Source: CAD feature listing. Evaluate the final solid. Frame: model axes, mm. A direction names the side the tool comes from. Round coordinates to 2 decimals unless told otherwise and drop trailing zeros. Order: outer loops, then holes, each group sorted by start corner. A loop starts at its lowest first (then second) coordinate and runs counter-clockwise, first axis right, second up. Notation, with made-up numbers: M 77.25,4.25 L 128.25,4.25 A21 ccw 128.25,10.25 Z; hole C -28.75,-28 d2. An arc over 180 degrees is marked long. Use one line per item in the form item = value. Start each with the question number.
Q1. Pull-direction query (Y, two-part tool) for faces 6 (the flat face through (0, -23.749, 3)), 7 (the flat face through (0, 28, 1.705)), 8 (the flat face through (4, 1, 2.54)); classes: pulls with the +Y half, pulls with the -Y half, needs draft (parallel to the pull), parting line crosses it, or undercut.
Q2. Contact query for flat-ended pins moving along their axis: pin 1 (2 mm diameter, centred on y = 26, z = 2.5, fed in from +X); pin 2 (2 mm diameter, centred on y = 26, z = 3.5, fed in from -X); pin 3 (2.5 mm diameter, centred on x = -2.5, y = 26, fed in from -Z) (3 decimals). Output: stop coordinate, or through.
Q3. Section B-B (z = 1). Return the cut outline in (x, y).
Q4. Section A-A (y = 4). Return the cut outline in (x, z), plus the area to 3 significant figures.
Q5. Reachability of faces 1 (the flat face through (0, 28, 4.245)), 2 (the flat face through (-5.156, 5.202, 4.269)), 3 (the flat face through (5.08, 28, 3)), 4 (the flat face through (0, 0, 0)), 5 (the flat face through (-5.08, 28, 3)) from +Z, -Z, +X, -X, +Y, -Y: full face, straight path, thin tool, end or side. Return the list, or none.
Q6. Material intervals for probe 1 along Y at (x, z) = (3.5, 5.1); probe 2 along Y at (x, z) = (1.75, 3.8); probe 3 along Y at (x, z) = (5.75, 4.95), sorted ascending.
from build123d import *

# Parameters (mm, degrees)
SKETCH1_W           = 17.38
SKETCH1_H           = 47.498
BOSS_EXTRUDE1_DEPTH = 5.95
CUT_EXTRUDE1_DEPTH  = 3.41
SKETCH3_W           = 10.16
SKETCH3_H           = 2.54
BOSS_EXTRUDE2_DEPTH = 7.62


with BuildPart() as part:
    # Sketch1 → Boss-Extrude1 (new body)
    with BuildSketch(Plane.XY):
        Rectangle(SKETCH1_W, SKETCH1_H)
    extrude(amount=BOSS_EXTRUDE1_DEPTH)

    # Sketch2 → Cut-Extrude1 (cut)
    with BuildSketch(Plane.XY.offset(5.95)):
        with BuildLine():
            Line((7.442756003, 9.924455156), (7.491268126, 9.618455606))
            add(Edge.make_bspline(
                [(7.491268126, 9.618455606), (7.388196446, 9.466942554), (7.190794115, 9.176765567), (6.883635039, 8.77416687), (6.580334345, 8.424256906), (6.271574884, 8.117843462), (5.940370317, 7.841299159), (5.568441188, 7.578876003), (5.153754118, 7.310436522), (4.852926765, 7.147246701), (4.696223459, 7.062239856)],
                knots=[0, 0, 0, 0, 1.145964768, 2.194745584, 3.165202406, 4.03990847, 4.912501504, 5.860303535, 6.885415487, 8, 8, 8, 8], degree=3))
            add(Edge.make_bspline(
                [(4.696223459, 7.062239856), (4.499744398, 6.967232704), (4.102902364, 6.775340341), (3.474153814, 6.538191996), (2.813554004, 6.333237061), (2.120776353, 6.162580703), (1.399657714, 6.026815112), (0.651510405, 5.937381635), (-0.120298453, 5.873381172), (-0.643704604, 5.867395245), (-0.908792682, 5.86436357)],
                knots=[0, 0, 0, 0, 0.905325806, 1.828547692, 2.785348579, 3.774441141, 4.787925238, 5.828395329, 6.90015334, 8, 8, 8, 8], degree=3))
            add(Edge.make_bspline(
                [(-0.908792682, 5.86436357), (-1.183775776, 5.868319524), (-1.744155055, 5.876381236), (-2.60042752, 5.931891418), (-3.488027549, 6.016072254), (-4.088461448, 6.098524731), (-4.394202187, 6.140509505)],
                knots=[0, 0, 0, 0, 0.943008224, 1.921726389, 2.941743778, 4, 4, 4, 4], degree=3))
            Line((-4.394202187, 6.140509505), (-5.245030203, 1.177346077))
            add(Edge.make_bspline(
                [(-5.245030203, 1.177346077), (-5.099692133, 1.252367706), (-4.817426132, 1.398069757), (-4.4023402, 1.604243124), (-4.006704111, 1.790847965), (-3.632644493, 1.958676402), (-3.278177346, 2.103991861), (-2.947838119, 2.237174313), (-2.634386649, 2.343936776), (-2.239987634, 2.466535927), (-1.735943769, 2.588441657), (-1.096664304, 2.685171937), (-0.408909829, 2.752005624), (0.066252368, 2.757006699), (0.311473815, 2.759587651)],
                knots=[0, 0, 0, 0, 1.006594111, 1.95494061, 2.852161939, 3.698632082, 4.47771994, 5.20984462, 5.890144692, 6.514895121, 7.751501423, 9.076797217, 10.491395109, 12, 12, 12, 12], degree=3))
            add(Edge.make_bspline(
                [(0.311473815, 2.759587651), (0.535398839, 2.755977577), (0.974846729, 2.748892886), (1.620475428, 2.715284292), (2.237431508, 2.640791764), (2.828133868, 2.549610207), (3.391581711, 2.431161677), (3.926410539, 2.283829718), (4.436803767, 2.118613947), (4.916396667, 1.918999578), (5.371826845, 1.701125088), (5.793685602, 1.447774573), (6.191678015, 1.175540089), (6.432055206, 0.966979497), (6.550879266, 0.863883124)],
                knots=[0, 0, 0, 0, 1.209491551, 2.373600323, 3.489351857, 4.563959151, 5.600865615, 6.596587735, 7.558914106, 8.495791867, 9.400120309, 10.282627716, 11.15106276, 12, 12, 12, 12], degree=3))
            add(Edge.make_bspline(
                [(6.550879266, 0.863883124), (6.663701743, 0.742591932), (6.887885733, 0.501580172), (7.185905623, 0.107991252), (7.434808919, -0.317506707), (7.64735089, -0.762667624), (7.815411217, -1.223810977), (7.933572717, -1.692856119), (8.013981471, -2.164737406), (8.021265636, -2.481883253), (8.024901487, -2.64018489)],
                knots=[0, 0, 0, 0, 1.019710416, 2.026216391, 3.032489163, 4.05009723, 5.060530396, 6.048889042, 7.026113504, 8, 8, 8, 8], degree=3))
            add(Edge.make_bspline(
                [(8.024901487, -2.64018489), (8.020801767, -2.804619839), (8.012753023, -3.127445431), (7.943075826, -3.602494497), (7.831393213, -4.057156952), (7.67809346, -4.496086456), (7.475268481, -4.912593105), (7.231250027, -5.312871427), (6.938962553, -5.690361738), (6.716016962, -5.922311768), (6.603123092, -6.039765252)],
                knots=[0, 0, 0, 0, 1.041176999, 2.04408236, 3.034027167, 4.003470328, 4.983202096, 5.962965549, 6.968498547, 8, 8, 8, 8], degree=3))
            add(Edge.make_bspline(
                [(6.603123092, -6.039765252), (6.405699461, -6.215392151), (6.007486189, -6.569640332), (5.32662517, -7.011218259), (4.58377472, -7.392320821), (3.766799238, -7.694680543), (2.886211455, -7.939522552), (1.934509396, -8.101388624), (0.917305834, -8.210370201), (0.214760817, -8.221040232), (-0.14752551, -8.226542522)],
                knots=[0, 0, 0, 0, 0.871069273, 1.756990004, 2.669566264, 3.621983655, 4.627000268, 5.682036848, 6.804679652, 8, 8, 8, 8], degree=3))
            add(Edge.make_bspline(
                [(-0.14752551, -8.226542522), (-0.370250634, -8.222244049), (-0.816200421, -8.213637462), (-1.482946375, -8.166140654), (-2.145331954, -8.078795756), (-2.791605268, -7.961417463), (-3.403604951, -7.819259345), (-3.958712163, -7.654815969), (-4.453900955, -7.481257394), (-4.749947343, -7.333786701), (-4.890518529, -7.263763451)],
                knots=[0, 0, 0, 0, 1.095684565, 2.19382659, 3.285951729, 4.380508114, 5.423877159, 6.374492448, 7.228163105, 8, 8, 8, 8], degree=3))
            add(Edge.make_bspline(
                [(-4.890518529, -7.263763451), (-5.035629193, -7.182452627), (-5.316509414, -7.025065144), (-5.694035748, -6.740579878), (-6.019519859, -6.431088542), (-6.295032988, -6.097913353), (-6.51309252, -5.744206053), (-6.667017422, -5.373777783), (-6.766809982, -4.991418752), (-6.777243361, -4.730546951), (-6.782491355, -4.599328348)],
                knots=[0, 0, 0, 0, 1.160681474, 2.246647206, 3.291271732, 4.291304077, 5.25829909, 6.181203858, 7.085144929, 8, 8, 8, 8], degree=3))
            add(Edge.make_bspline(
                [(-6.782491355, -4.599328348), (-6.774342349, -4.453081073), (-6.75846843, -4.168197538), (-6.64211866, -3.759871717), (-6.436538728, -3.397764213), (-6.163895247, -3.081023671), (-5.833430689, -2.820020292), (-5.457625005, -2.631179544), (-5.044250192, -2.513816473), (-4.755734581, -2.501171297), (-4.606909191, -2.494648518)],
                knots=[0, 0, 0, 0, 1.038363749, 2.022688871, 2.983899271, 3.973918752, 4.974410771, 5.954403577, 6.944817285, 8, 8, 8, 8], degree=3))
            add(Edge.make_bspline(
                [(-4.606909191, -2.494648518), (-4.507163048, -2.496981892), (-4.312628946, -2.501532653), (-4.031008634, -2.552467514), (-3.765664982, -2.629947355), (-3.520661715, -2.74257489), (-3.294573312, -2.881087206), (-3.092603306, -3.045610231), (-2.914473539, -3.235149346), (-2.763280777, -3.446234353), (-2.638351732, -3.674894842), (-2.548205754, -3.918478563), (-2.494918861, -4.17535582), (-2.487384773, -4.350303052), (-2.483570852, -4.438865169)],
                knots=[0, 0, 0, 0, 1.117637543, 2.179719547, 3.199437565, 4.211008827, 5.194574363, 6.166491412, 7.123978993, 8.103677089, 9.071378429, 10.038174012, 11.006880757, 12, 12, 12, 12], degree=3))
            add(Edge.make_bspline(
                [(-2.483570852, -4.438865169), (-2.486995627, -4.527517151), (-2.493771023, -4.70290165), (-2.552315647, -4.956438553), (-2.640742431, -5.197727564), (-2.776563998, -5.418114374), (-2.939315934, -5.629950077), (-3.146823442, -5.820016584), (-3.384493352, -6.001663071), (-3.565500253, -6.100586139), (-3.659056927, -6.151716307)],
                knots=[0, 0, 0, 0, 0.968529955, 1.916089601, 2.833465673, 3.766948701, 4.736052034, 5.746774587, 6.835379905, 8, 8, 8, 8], degree=3))
            add(Edge.make_bspline(
                [(-3.659056927, -6.151716307), (-3.712593015, -6.195118685), (-3.810012219, -6.274097656), (-3.926920197, -6.402182193), (-4.001195782, -6.530313333), (-4.012238567, -6.618709273), (-4.017300302, -6.659227755)],
                knots=[0, 0, 0, 0, 1.288779764, 2.34518258, 3.241473203, 4, 4, 4, 4], degree=3))
            add(Edge.make_bspline(
                [(-4.017300302, -6.659227755), (-4.014862106, -6.693558852), (-4.009786068, -6.765032163), (-3.94889938, -6.86383505), (-3.865505152, -6.962509198), (-3.747621078, -7.0590999), (-3.59734133, -7.150700716), (-3.414668231, -7.240893328), (-3.200044936, -7.328812331), (-2.867030136, -7.443506304), (-2.414722193, -7.569316413), (-1.839757858, -7.670449008), (-1.236208093, -7.736106558), (-0.824385614, -7.744563892), (-0.613988238, -7.748884688)],
                knots=[0, 0, 0, 0, 0.326627239, 0.679999541, 1.087570525, 1.571741335, 2.136209263, 2.778409567, 3.529552134, 4.365937735, 6.165921372, 8.039005593, 9.976354196, 12, 12, 12, 12], degree=3))
            add(Edge.make_bspline(
                [(-0.613988238, -7.748884688), (-0.42349165, -7.745898893), (-0.053933814, -7.740106537), (0.480092866, -7.67864014), (0.976569924, -7.583764599), (1.432246926, -7.446925264), (1.848139012, -7.268810492), (2.227817186, -7.057803498), (2.567389934, -6.802022096), (2.864540024, -6.502050413), (3.12901858, -6.16407249), (3.352639163, -5.778648178), (3.54280588, -5.350498704), (3.699090595, -4.879386484), (3.817527637, -4.363147203), (3.901267526, -3.80421506), (3.954403228, -3.199710621), (3.96125619, -2.7821062), (3.964809902, -2.565550853)],
                knots=[0, 0, 0, 0, 1.145984371, 2.223176321, 3.230327741, 4.184709763, 5.080198491, 5.948392179, 6.792829292, 7.629197606, 8.482744051, 9.368637587, 10.303560962, 11.297831961, 12.351033038, 13.487071465, 14.696881343, 16, 16, 16, 16], degree=3))
            add(Edge.make_bspline(
                [(3.964809902, -2.565550853), (3.959937282, -2.315186172), (3.95054273, -1.832475769), (3.854905269, -1.138827256), (3.705638698, -0.502736617), (3.487857452, 0.072698671), (3.212336232, 0.590456281), (2.869977731, 1.042931556), (2.464404193, 1.430095093), (1.998885296, 1.746615006), (1.483054716, 1.997270407), (0.925314836, 2.181919986), (0.322799369, 2.28608044), (-0.091155302, 2.300584907), (-0.304256986, 2.308051731)],
                knots=[0, 0, 0, 0, 1.224131662, 2.360161531, 3.418424534, 4.414143726, 5.361687872, 6.278160415, 7.177748908, 8.092603741, 9.020660508, 9.975155306, 10.957620613, 12, 12, 12, 12], degree=3))
            add(Edge.make_bspline(
                [(-0.304256986, 2.308051731), (-0.585965965, 2.299911613), (-1.136361477, 2.284007669), (-1.811836605, 2.167686698), (-2.337007345, 2.039517007), (-2.732310337, 1.908362031), (-3.140497373, 1.762367668), (-3.553566201, 1.578877843), (-3.981742925, 1.379844177), (-4.417153582, 1.143324516), (-4.874022359, 0.893907905), (-5.176248262, 0.706169561), (-5.330859345, 0.6101274)],
                knots=[0, 0, 0, 0, 1.569199768, 3.065860781, 3.809147302, 4.580990623, 5.38603441, 6.224540817, 7.099163695, 8.017256459, 8.985678849, 10, 10, 10, 10], degree=3))
            Line((-5.330859345, 0.6101274), (-5.827175687, 0.6101274))
            Line((-5.827175687, 0.6101274), (-4.465104521, 9.924455156))
            add(Edge.make_bspline(
                [(-4.465104521, 9.924455156), (-4.315984039, 9.880431687), (-4.028541468, 9.795572662), (-3.610488685, 9.680706455), (-3.217546123, 9.59555299), (-2.963853205, 9.550545578), (-2.841814227, 9.528894762)],
                knots=[0, 0, 0, 0, 1.115879267, 2.150953381, 3.110516124, 4, 4, 4, 4], degree=3))
            add(Edge.make_bspline(
                [(-2.841814227, 9.528894762), (-2.510146411, 9.477884697), (-1.830201619, 9.373310099), (-0.775608412, 9.285032005), (0.332929285, 9.21530606), (1.09127166, 9.210452917), (1.479496486, 9.207968405)],
                knots=[0, 0, 0, 0, 0.928037139, 1.90254824, 2.926233227, 4, 4, 4, 4], degree=3))
            add(Edge.make_bspline(
                [(1.479496486, 9.207968405), (1.857705195, 9.211620808), (2.587136827, 9.218665008), (3.650367069, 9.270738299), (4.655930506, 9.361259539), (5.618408289, 9.504787441), (6.545008139, 9.689890411), (7.146144347, 9.846956071), (7.442756003, 9.924455156)],
                knots=[0, 0, 0, 0, 1.129737635, 2.178866713, 3.179008279, 4.144335706, 5.084381125, 6, 6, 6, 6], degree=3))
        make_face()
    extrude(amount=-CUT_EXTRUDE1_DEPTH, mode=Mode.SUBTRACT)

    # Sketch3 → Boss-Extrude2 (add)
    with BuildSketch(Plane(origin=(0, 23.749, 0), x_dir=(1, 0, 0), z_dir=(0, 1, 0))):
        with Locations((0, -2.975)):
            Rectangle(SKETCH3_W, SKETCH3_H)
    extrude(amount=BOSS_EXTRUDE2_DEPTH)


solid = part.part
Results list:
q1.face_6 = pulls with the -Y half
q1.face_7 = needs draft
q1.face_8 = undercut
q2.pin_1 = 5.08
q2.pin_2 = -5.08
q2.pin_3 = 1.705
q3.outline = M -8.69,-23.75 L 8.69,-23.75 L 8.69,23.75 L -8.69,23.75 Z
q4.outline = M -8.69,0 L 8.69,0 L 8.69,5.95 L -4.76,5.95 L -4.76,2.54 L -5.33,2.54 L -5.33,5.95 L -8.69,5.95 Z
q4.area = 101 mm2
q5.face_1 = +Z, +X, -X, +Y
q5.face_2 = +Z
q5.face_3 = +Z, -Z, +X, +Y
q5.face_4 = -Z, +X, -X, +Y, -Y
q5.face_5 = +Z, -Z, -X, +Y
q6.probe_1 = -23.75 to -7.76, -5.44 to 0.01, 2.4 to 6.55, 9.27 to 23.75
q6.probe_2 = -23.75 to -8.12, -7.31 to 1.86, 2.7 to 6.09, 9.21 to 31.37
q6.probe_3 = -23.75 to -6.73, 1.47 to 7.71, 9.54 to 23.75
